Can you work these out from the model? Positions are in its coordinate system, mm. A direction names the side the tool comes from. Round coordinates to 2 decimals unless told otherwise and drop trailing zeros. Loops run counter-clockwise (first coordinate to the right, second up) from the corner with the lowest first, then second, coordinate; pieces in that order, holes last. Notation, with made-up numbers: M 82.25,-38.5 L 98.25,-38.5 A12 ccw 98.25,-33.5 Z; hole C 76.25,30.5 d11. An arc over 180 degrees is marked long. Use a Markdown table: item, result. Add a question column.
```python
from build123d import *

# Parameters (mm, degrees)
F1_DEPTH = 40
F0_R     = 10
F2_DEPTH = 10


with BuildPart() as f1:
    # F0 (on Front) → F1 (new body)
    with BuildSketch(Plane.XZ):
        with BuildLine():
            ThreePointArc((-85, 0), (-93.75, 23.150324), (-115.625, 34.725486))
            ThreePointArc((-115.625, 34.725486), (-155, 0), (-115.625, -34.725486))
            ThreePointArc((-115.625, -34.725486), (-93.75, -23.150324), (-85, 0))
        make_face()
        with BuildLine():
            ThreePointArc((-111.339746, -5), (-130, 0), (-111.339746, 5))
            Line((-111.339746, 5), (-108, 5))
            Line((-108, 5), (-108, -5))
            Line((-108, -5), (-111.339746, -5))
        make_face(mode=Mode.SUBTRACT)
    extrude(amount=F1_DEPTH)

    # F0 (on Front) → F2 (join)
    with BuildSketch(Plane.XZ):
        with BuildLine():
            ThreePointArc((2.5, -19.843135), (15, -13.228757), (20, 0))
            ThreePointArc((20, 0), (15, 13.228757), (2.5, 19.843135))
            ThreePointArc((2.5, 19.843135), (-20, 0), (2.5, -19.843135))
        make_face()
        Circle(F0_R, mode=Mode.SUBTRACT)
        with BuildLine():
            ThreePointArc((2.5, -19.843135), (-20, 0), (2.5, 19.843135))
            Line((2.5, 19.843135), (-115.625, 34.725486))
            ThreePointArc((-115.625, 34.725486), (-93.75, 23.150324), (-85, 0))
            ThreePointArc((-85, 0), (-93.75, -23.150324), (-115.625, -34.725486))
            Line((-115.625, -34.725486), (2.5, -19.843135))
        make_face()
        with BuildLine():
            ThreePointArc((-85, 0), (-93.75, 23.150324), (-115.625, 34.725486))
            ThreePointArc((-115.625, 34.725486), (-155, 0), (-115.625, -34.725486))
            ThreePointArc((-115.625, -34.725486), (-93.75, -23.150324), (-85, 0))
        make_face()
        with BuildLine():
            ThreePointArc((-111.339746, -5), (-130, 0), (-111.339746, 5))
            Line((-111.339746, 5), (-108, 5))
            Line((-108, 5), (-108, -5))
            Line((-108, -5), (-111.339746, -5))
        make_face(mode=Mode.SUBTRACT)
    extrude(amount=F2_DEPTH)


solid = f1.part
```
(1) If I drill on probe 1 along Z at (x, y) = (-120, -17); probe 2 along X at (y, z) = (-23.5, -0.5); probe 3 along X at (y, z) = (-5.5, 9), over which ranges is the centre line in solid material (lowest first)? Write a range as [from, to].
(2) On a 3-axis mill with a long thin cutter (end or side, diameter ignored), from which of +Z, -Z, +X, -X, +Y, -Y can I reach the whole of each face in a straight line? I mean faces 5 (the face through (-110, -20, 5)), 6 (the face through (-112.7, -40, -7.3)). Say none if no direction works.
(3) Suppose I cut it at A-A on x = -120. List the corners of the cut face in (y, z) for me.
(4) Suppose I cut it at C-C on y = -27. List the corners of the cut face in (x, z) for me (3 decimals), and give its area (3 significant figures).
(5) I'm going to push flat-ended pins straight in: pin 1 (3 mm diameter, centred on y = -17.5, z = 2, fed in from -X); pin 2 (12 mm diameter, centred on x = -73.5, y = -15, fed in from -Z); pin 3 (2 mm diameter, centred on x = -24.5, z = -3.5, fed in from -Y); pin 4 (18 mm diameter, centred on x = -120, z = 0, fed in from -Y). Where does each tip first touch, or does it pass through?
(6) Thinking about a two-plate mould opening in X: for faces 1 (the face through (-110, -20, -5)), 2 (the face through (-55.74, -4.93, 27.18)), 3 (the face through (-108, -20, 0)), 4 (the face through (-69, 0, 0)), which applies, released by +X, released by -X, zero draft, split by the parting line, or undercut?
(7) Suppose I cut it at D-D on z = -23. List the corners of the cut face in (x, y) for me.
(8) Suppose I cut it at B-B on y = -7. List the corners of the cut face in (x, z) for me (3 decimals).
Results below:
| question | item | result |
|---|---|---|
| 1 | probe 1 | z = [-35, -10], [10, 35] |
| 1 | probe 2 | x = [-155, -129.99], [-108, -85] |
| 1 | probe 3 | x = [-153.82, -124.36], [-115.64, -4.36], [4.36, 17.86] |
| 2 | face 5 | +Y, -Y |
| 2 | face 6 | +Z, -Z, +X, -X, -Y |
| 3 | outline | M -40,-35 L 0,-35 L 0,-10 L -40,-10 Z; M -40,10 L 0,10 L 0,35 L -40,35 Z |
| 4 | outline | C -120,0 d70; hole M -111.34,-5 L -108,-5 L -108,5 L -111.34,5 A10 ccw long Z |
| 4 | area | 3,510 mm² |
| 5 | pin 1 | stops at x = -155 |
| 5 | pin 2 | stops at z = -29.84 |
| 5 | pin 3 | stops at y = -10 |
| 5 | pin 4 | passes through |
| 6 | face 1 | undercut |
| 6 | face 2 | released by +X |
| 6 | face 3 | undercut |
| 6 | face 4 | zero draft |
| 7 | outline | M -146.38,-40 L -93.62,-40 L -93.62,-10 L -22.56,-10 L -22.56,0 L -146.38,0 Z |
| 8 | outline | M -115.625,-34.725 L 2.5,-19.843 A20 ccw 20,0 A20 ccw 2.5,19.843 L -115.625,34.725 A35 ccw long Z; hole M -111.34,-5 L -108,-5 L -108,5 L -111.34,5 A10 ccw long Z; hole C 0,0 d20 |
